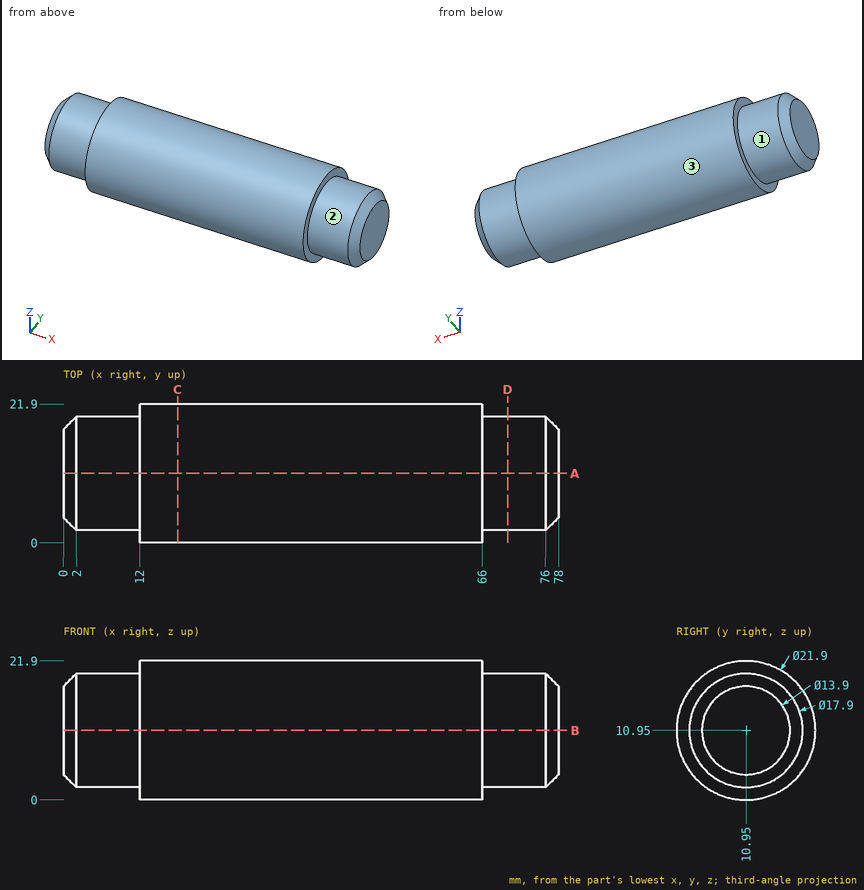
Could you check a few things on this drawing? It's one solid part, dimensions in mm from its lowest x, y, z. A direction names the side the tool comes from. Give positions to 0.01 mm unless a question says otherwise; leave off trailing zeros. Loops run counter-clockwise (first coordinate to the right, second up) from the corner with the lowest first, then second, coordinate; pieces in that order, holes last. Notation, with made-up numbers: M -20,-33 L 20,-33 A29 ccw 20,-6 Z; hole C -22.5,30 d9. An arc over 180 degrees is marked long. Answer as a JSON object with one key per item and string values.
Q1. Suppose I cut it at D-D, the plane x = 70. List the corners of the cut face in (y, z) for me.
Values found:
{"outline": "C 10.95,10.95 d17.9"}
Q2. For P1, Ø1.5, axis at x = 21.5, z = 14, coming from the +Y side; P2, Ø1, axis at x = 60.5, z = 18.5, coming from the +Y side; P3, Ø5, axis at x = 16, y = 18.5, coming from the -Z side; P4, Ø3, axis at y = 7.5, z = 16.5, coming from the -X side, each with a flat end and sliding along its axis, tell me the tip position at first contact or that it passes through.
Values found:
{"P1": "stops at y = 21.66", "P2": "stops at y = 19.33", "P3": "stops at z = 1.23", "P4": "stops at x = 0"}
Q3. Suppose I cut it at C-C, the plane x = 18. List the corners of the cut face in (y, z) for me, plus the area to 3 significant figures.
Values found:
{"outline": "C 10.95,10.95 d21.9", "area": "377 mm²"}
Q4. For the marked faces 1, 2 and 3, which set-ups out of +Z, -Z, +X, -X, +Y, -Y let a thin tool reach every point of the face, with its end or its side?
Values found:
{"face 1": "-X", "face 2": "+X", "face 3": "+X, -X"}
Q5. Suppose I cut it at A-A, the plane y = 10.95. List the corners of the cut face in (x, z) for me, plus the area to 3 significant figures.
Values found:
{"outline": "M 0,4 L 2,2 L 12,2 L 12,0 L 66,0 L 66,2 L 76,2 L 78,4 L 78,17.9 L 76,19.9 L 66,19.9 L 66,21.9 L 12,21.9 L 12,19.9 L 2,19.9 L 0,17.9 Z", "area": "1,600 mm²"}
Q6. If I drill on probe 1 along X at (y, z) = (21, 11); probe 2 along Y at (x, z) = (24, 4.25); probe 3 along Y at (x, z) = (4.5, 7.5), over which ranges is the centre line in solid material (lowest first)? Write a range as [from, to].
Values found:
{"probe 1": "x = [12, 66]", "probe 2": "y = [2.29, 19.61]", "probe 3": "y = [2.69, 19.21]"}
